Could you check a few things on this model? Use its own coordinates, in mm. A direction names the side the tool comes from. Round coordinates to 2 decimals unless told otherwise and drop trailing zeros. Loops run counter-clockwise (first coordinate to the right, second up) from the corner with the lowest first, then second, coordinate; pieces in that order, holes last. Notation, with made-up numbers: M 75,-39 L 89,-39 A21 cw 89,-11 Z; hole C 41,17.25 d8. An arc over 180 degrees is marked long. One line per item, written item: value. Start each with the question number.
Q1. Please list where these lines run through material, in increasing order: line 1 along X through (y, z) = (14.25, 0); line 2 along Y through (x, z) = (-4, 2); line 3 along Y through (x, z) = (-25, 14).
Q2. Which directions (+Z, -Z, +X, -X, +Y, -Y) give clear straight access to the entire face, cutting with the end or side of a thin tool? Please do faces 4 (the face through (8.25, -9.85, 26.18)), 5 (the face through (-8.741, 10.367, -27.756)), 6 (the face through (29.384, 10.353, 6.525)).
Q3. Imagine slicing it at C-C (z = 0). Please give me the cut outline in (x, y).
Q4. Imagine slicing it at A-A (x = 0). Please give me the cut outline in (y, z), then the cut area to 4 significant figures.
Q5. Imagine slicing it at D-D (y = 9.5). Please give me the cut outline in (x, z).
Q6. Imagine slicing it at B-B (y = -3). Please give me the cut outline in (x, z).
Q7. I'm going to push flat-ended pins straight in: pin 1 Ø5 at (y, z) = (-13, -11.5) entering from -X; pin 2 Ø18 at (x, z) = (12.5, -13.5) entering from -Y; pin 3 Ø6 at (x, y) = (-7, -14) entering from +Z. Where does each tip first touch, or does it pass through?
Q8. Thinking about a two-plate mould opening in Z: for faces 1 (the face through (0, 21, 0)), 2 (the face through (-27.773, -10.353, -6.167)), 3 (the face through (0, 20, 0)), which applies, released by +Z, released by -Z, zero draft, split by the parting line, or undercut?
from build123d import *

# Parameters (mm, degrees)
SKETCH1_R           = 30.1
BOSS_EXTRUDE1_DEPTH = 21
SKETCH1_3_R         = 28.45
BOSS_EXTRUDE2_DEPTH = 21
SHELL1_T            = -1


with BuildPart() as part:
    # Sketch1 → Boss-Extrude1 (new body)
    with BuildSketch(Plane(origin=(0, 0, 0), x_dir=(1, 0, 0), z_dir=(0, 1, 0))):
        with Locations(Location((0, 0, 0), (0, 0, 90))):
            Circle(SKETCH1_R)
    extrude(amount=BOSS_EXTRUDE1_DEPTH)

    # Sketch1_3 → Boss-Extrude2 (add)
    with BuildSketch(Plane(origin=(0, 0, 0), x_dir=(1, 0, 0), z_dir=(0, 1, 0))):
        with Locations(Location((0, 0, 0), (0, 0, 270))):
            Circle(SKETCH1_3_R)
    extrude(amount=-BOSS_EXTRUDE2_DEPTH)

    # Shell1
    shell1_openings = [part.faces().sort_by_distance(p)[0] for p in [
        (0, -21, 0),
    ]]
    offset(amount=SHELL1_T, openings=shell1_openings, kind=Kind.INTERSECTION)


solid = part.part
Report:
1. line 1: x = -30.1 to -29.1, 29.1 to 30.1
1. line 2: y = 20 to 21
1. line 3: y = 0 to 1, 20 to 21
2. face 4: -Y
2. face 5: none
2. face 6: +Y, -Y
3. outline: M -30.1,0 L -28.45,0 L -28.45,-21 L -27.45,-21 L -27.45,1 L -29.1,1 L -29.1,20 L 29.1,20 L 29.1,1 L 27.45,1 L 27.45,-21 L 28.45,-21 L 28.45,0 L 30.1,0 L 30.1,21 L -30.1,21 Z
4. outline: M -21,-28.45 L 0,-28.45 L 0,-30.1 L 21,-30.1 L 21,30.1 L 0,30.1 L 0,28.45 L -21,28.45 L -21,27.45 L 1,27.45 L 1,29.1 L 20,29.1 L 20,-29.1 L 1,-29.1 L 1,-27.45 L -21,-27.45 Z
4. area: 145.5 mm²
5. outline: C 0,0 d60.2; hole C 0,0 d58.2
6. outline: C 0,0 d56.9; hole C 0,0 d54.9
7. pin 1: stops at x = -26.99
7. pin 2: stops at y = 20
7. pin 3: stops at z = 28.17
8. face 1: zero draft
8. face 2: split by the parting line
8. face 3: undercut
